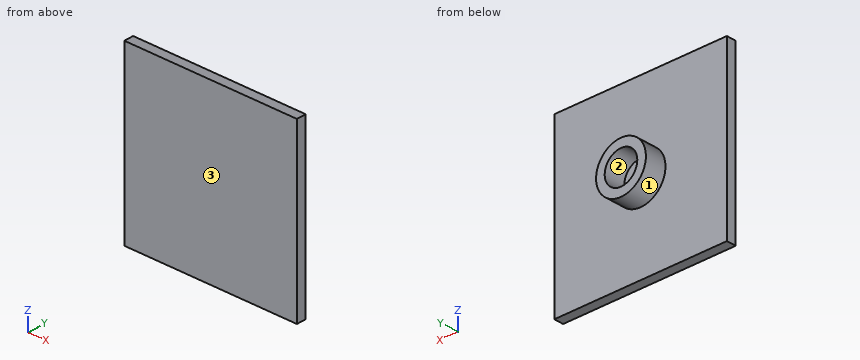
```python
from build123d import *

# Parameters (mm, degrees)
SKETCH1_W           = 114.3
SKETCH1_H           = 114.3
BOSS_EXTRUDE1_DEPTH = 6.35
SKETCH2_R           = 16.51
BOSS_EXTRUDE2_DEPTH = 14
SKETCH3_R           = 10.8
CUT_EXTRUDE1_DEPTH  = 14


with BuildPart() as part:
    # Sketch1 → Boss-Extrude1 (new body)
    with BuildSketch(Plane(origin=(0, 0, 0), x_dir=(1, 0, 0), z_dir=(0, 1, 0))):
        with Locations((57.15, 57.15)):
            Rectangle(SKETCH1_W, SKETCH1_H)
    extrude(amount=BOSS_EXTRUDE1_DEPTH)

    # Sketch2 → Boss-Extrude2 (add)
    with BuildSketch(Plane(origin=(0, 6.35, 0), x_dir=(1, 0, 0), z_dir=(0, 1, 0))):
        with Locations(Location((57.15, 57.15, 0), (0, 0, 270))):
            Circle(SKETCH2_R)
    extrude(amount=BOSS_EXTRUDE2_DEPTH)

    # Sketch3 → Cut-Extrude1 (cut)
    with BuildSketch(Plane(origin=(0, 20.35, 0), x_dir=(1, 0, 0), z_dir=(0, 1, 0))):
        with Locations(Location((57.15, 57.15, 0), (0, 0, 270))):
            Circle(SKETCH3_R)
    extrude(amount=-CUT_EXTRUDE1_DEPTH, mode=Mode.SUBTRACT)


solid = part.part
```
The model under review builds one solid part; all positions refer to its coordinate system, in mm. Face numbers are marked on the shaded views. Round coordinates to 2 decimals unless told otherwise and drop trailing zeros. Loops run counter-clockwise (first coordinate to the right, second up) from the corner with the lowest first, then second, coordinate; pieces in that order, holes last.
1) The part is to be moulded in two halves that separate along Z. For the marked faces 1, 2 and 3, say which applies: pulls with the +Z half, pulls with the -Z half, needs draft (parallel to the pull), parting line crosses it, or undercut.
Values follow:
face 1: parting line crosses it
face 2: undercut
face 3: needs draft
2) Consider section C-C on z = -57.15. State the section outline as (x, y) points, then the cut area to 3 significant figures.
Values follow:
outline: (0, 0) - (114.3, 0) - (114.3, 6.35) - (73.66, 6.35) - (73.66, 20.35) - (67.95, 20.35) - (67.95, 6.35) - (46.35, 6.35) - (46.35, 20.35) - (40.64, 20.35) - (40.64, 6.35) - (0, 6.35) - close
area: 886 mm2
3) Wall thickness on line 1 along X through (y, z) = (14.75, -57.15); line 2 along Z through (x, y) = (56.5, 8.75); line 3 along Y through (x, z) = (48.5, -10.5): over which ranges is each line inside the solid? List them lowest first.
Values follow:
line 1: x = 40.64 to 46.35, 67.95 to 73.66
line 2: z = -73.65 to -67.93, -46.37 to -40.65
line 3: y = 0 to 6.35
4) Consider section A-A on x = 57.15. State the section outline as (y, z) points, then the cut area to 3 significant figures.
Values follow:
outline: (0, -114.3) - (6.35, -114.3) - (6.35, -73.66) - (20.35, -73.66) - (20.35, -67.95) - (6.35, -67.95) - (6.35, -46.35) - (20.35, -46.35) - (20.35, -40.64) - (6.35, -40.64) - (6.35, 0) - (0, 0) - close
area: 886 mm2
5) Consider section B-B on y = 10. State the section outline as (x, z) points.
Values follow:
outline: circle Ø33.02 at (57.15, -57.15); hole circle Ø21.6 at (57.15, -57.15)
6) Clearance check with flat-ended pins moving along their axes: P1, Ø1.5, axis at y = 7, z = -86, coming from the +X side; P2, Ø12, axis at x = 84.5, z = -20, coming from the +Y side; P3, Ø6, axis at x = 69, y = 10.5, coming from the +Z side; P4, Ø8, axis at y = 12, z = -38, coming from the -X side. State where each tip first meets the part, or that it passes through.
Values follow:
P1: stops at x = 114.3
P2: stops at y = 6.35
P3: stops at z = -43.21
P4: stops at x = 50.59
7) Consider section D-D on x = 75. State the section outline as (y, z) points.
Values follow:
outline: (0, -114.3) - (6.35, -114.3) - (6.35, 0) - (0, 0) - close
